Check sheet for the drawn part. Datum: minimum x, y, z corner. Units: mm. A direction names the side the tool comes from. Coordinates: 2 decimals unless noted, no trailing zeros. Loops run counter-clockwise (first coordinate to the right, second up) from the corner with the lowest first, then second, coordinate; pieces in that order, holes last.
Q1. Material ranges on probe 1 along X at (y, z) = (47.5, 12.5); probe 2 along Y at (x, z) = (20, 15); probe 3 along Y at (x, z) = (19.5, 37.5), recorded low to high.
Q2. Mould release check, pull along X, two halves, no side actions. Record for the marked faces 1, 2, 3 and 4: +X half, -X half, draft (parallel to the pull), parting line (faces both ways), or undercut.
Q3. Sectioned sample at A-A (y = 47.5). Enter the section's corners in (x, z), then the cut area to 3 significant figures.
Q4. Access from +Z, -Z, +X, -X, +Y, -Y to the whole of each face (thin tool, end or side, straight path). Record for the marked faces 5, 6, 7 and 8.
Q5. Sectioned sample at D-D (z = 29.5). Enter the section's corners in (x, y) (3 decimals).
Q6. Go/stop test with flat-tipped pins: P1, Ø8, axis at y = 29.5, z = 30.5, coming from the +X side; P2, Ø5, axis at y = 57, z = 34.5, coming from the -X side; P3, Ø15, axis at x = 45, z = 57.5, coming from the -Y side; P4, Ø3, axis at x = 11, y = 27, coming from the +Z side. Record where each tip stops, or that it passes through.
Q7. Sectioned sample at B-B (x = 20). Enter the section's corners in (y, z), then the cut area to 3 significant figures.
Q8. Sectioned sample at C-C (x = 5.5). Enter the section's corners in (y, z), then the cut area to 3 significant figures.
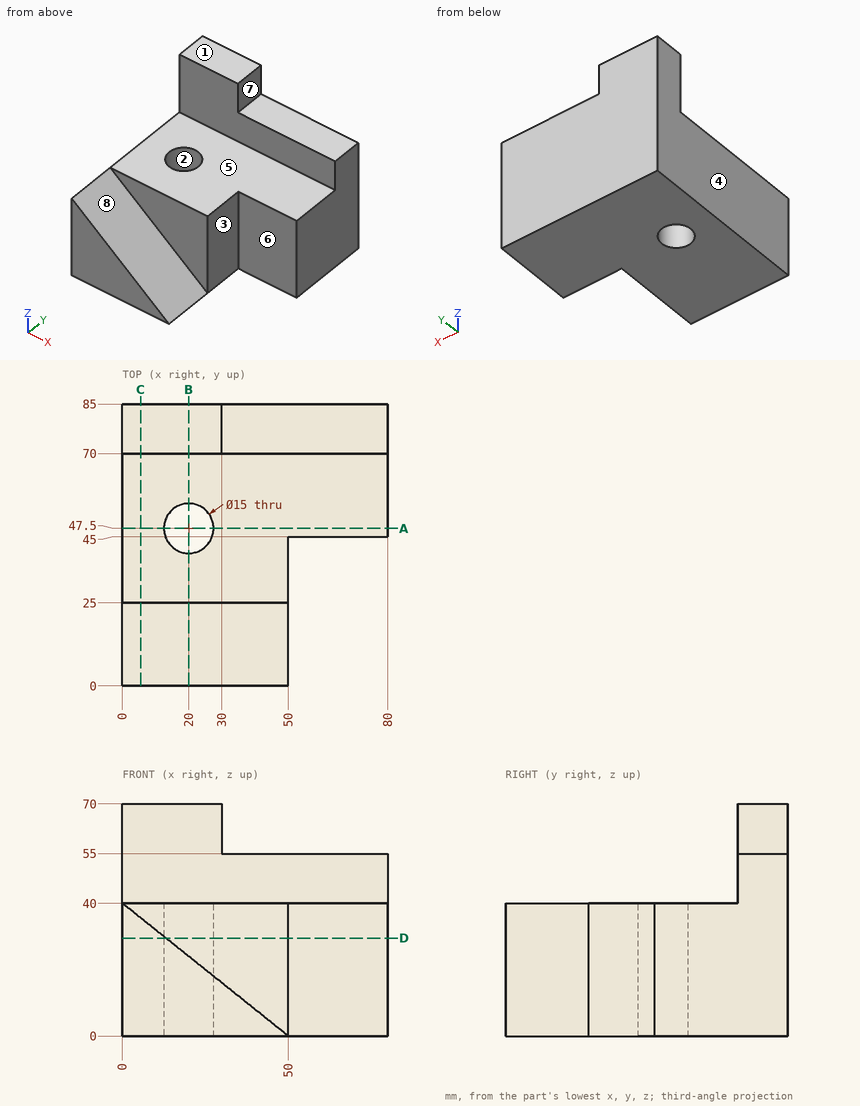
Geometry check:
1. probe 1: x = 0 to 12.5, 27.5 to 80
1. probe 2: y = 0 to 40, 55 to 85
1. probe 3: y = 25 to 40.02, 54.98 to 85
2. face 1: draft
2. face 2: undercut
2. face 3: +X half
2. face 4: -X half
3. outline: (0, 0) - (12.5, 0) - (12.5, 40) - (0, 40) - close; (27.5, 0) - (80, 0) - (80, 40) - (27.5, 40) - close
3. area: 2,600 mm2
4. face 5: +Z, +X, -X, -Y
4. face 6: +Z, -Z, +X, -Y
4. face 7: +Z, +X, +Y, -Y
4. face 8: +Z, +X, -Y
5. outline: (0, 0) - (13.125, 0) - (13.125, 25) - (50, 25) - (50, 45) - (80, 45) - (80, 85) - (0, 85) - close; hole circle Ø15 at (20, 47.5)
6. P1: stops at x = 50
6. P2: stops at x = 0
6. P3: stops at y = 70
6. P4: stops at z = 40
7. outline: (0, 0) - (40, 0) - (40, 40) - (25, 40) - (25, 24) - (0, 24) - close; (55, 0) - (85, 0) - (85, 70) - (70, 70) - (70, 40) - (55, 40) - close
7. area: 2,850 mm2
8. outline: (0, 0) - (85, 0) - (85, 70) - (70, 70) - (70, 40) - (25, 40) - (25, 35.6) - (0, 35.6) - close
8. area: 3,740 mm2
